Build history of the part. All positions in model axes, mm. Face numbers are marked on the shaded views. A direction names the side the tool comes from. Give positions to 0.01 mm unless a question says otherwise; leave off trailing zeros. Order: outer loops, then holes, each group sorted by start corner. A loop starts at its lowest first (then second) coordinate and runs counter-clockwise, first axis right, second up. Notation, with made-up numbers: (36.5, 1) - (72.5, 1) arc R31 ccw to (72.5, 25) - close; hole circle Ø6 at (-11, 30). An arc over 180 degrees is marked (long way). Answer in a Markdown table with one row per item.
```python
from build123d import *

# Parameters (mm, degrees)
F0_R     = 15
F1_DEPTH = 15
F3_DEPTH = 10
F4_R     = 6
F5_DEPTH = 10


with BuildPart() as f1:
    # F0 (on Top) → F1 (new body)
    with BuildSketch(Plane.XY):
        Circle(F0_R)
    extrude(amount=-F1_DEPTH)

    # F2 (on Top) → F3 (cut, symmetric)
    with BuildSketch(Plane.XY):
        Polygon((4.235221, 4.27539), (-15.764779, 4.27539), (-15.764779, 0.07539), (-0.001056, 0.035212), (-0.001056, -19.964788), (4.198944, -19.964788), align=None)
    extrude(amount=F3_DEPTH, both=True, mode=Mode.SUBTRACT)

    # F4 (on Top) → F5 (cut, symmetric)
    with BuildSketch(Plane.XY):
        with Locations((2.316362, 1.923726)):
            Circle(F4_R)
    extrude(amount=F5_DEPTH, both=True, mode=Mode.SUBTRACT)


solid = f1.part
```
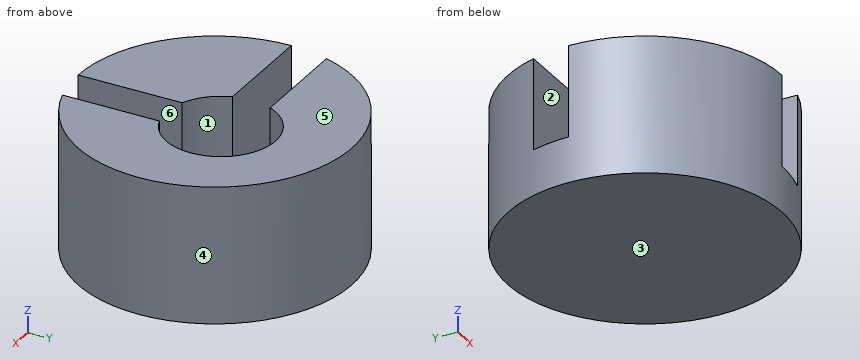
1. Drop flat-ended pins along their axis: P1, Ø1, axis at x = 10.5, y = 7, coming from the +Z side; P2, Ø5, axis at y = -7.5, z = -7, coming from the +X side; P3, Ø2, axis at y = 10.5, z = -12, coming from the -X side; P4, Ø1.5, axis at x = 10, z = -11, coming from the -Y side. Give the stop position or say it passes through.
Check result:
| item | result |
|---|---|
| P1 | stops at z = 0 |
| P2 | stops at x = 14.14 |
| P3 | stops at x = -11.61 |
| P4 | stops at y = -11.81 |
2. Cut at A-A on z = -7.25. Write the cut outline in (x, y).
Check result:
| item | result |
|---|---|
| outline | (-15, 0.07) arc R15 ccw to (0, -15) - (0, -3.61) arc R6 cw to (-3.38, 0.04) - close; (-14.38, 4.28) - (-3.2, 4.28) arc R6 cw (long way) to (4.22, -3.77) - (4.21, -14.4) arc R15 ccw (long way) to start |
3. Two-plate mould, pull along X, no slides. Class the marked faces 4, 5 and 6: +X half, -X half, draft (parallel to the pull), parting line (faces both ways), or undercut.
Check result:
| item | result |
|---|---|
| face 4 | parting line |
| face 5 | draft |
| face 6 | undercut |
4. Cut at B-B on x = -5. Write the cut outline in (y, z), and give its area (3 significant figures).
Check result:
| item | result |
|---|---|
| outline | (-14.14, -15) - (14.14, -15) - (14.14, 0) - (4.28, 0) - (4.28, -10) - (0.05, -10) - (0.05, 0) - (-14.14, 0) - close |
| area | 382 mm² |
5. Cut at C-C on y = -13. Write the cut outline in (x, z), and give its area (3 significant figures).
Check result:
| item | result |
|---|---|
| outline | (-7.48, -15) - (7.48, -15) - (7.48, 0) - (4.21, 0) - (4.21, -10) - (0, -10) - (0, 0) - (-7.48, 0) - close |
| area | 182 mm² |
6. Which spindle directions (+Z, -Z, +X, -X, +Y, -Y) get a long thin tool onto all of the face, cutting with end or side? Do the marked faces 1, 2 and 3. Say none if no direction does.
Check result:
| item | result |
|---|---|
| face 1 | +Z |
| face 2 | +Z, -X |
| face 3 | -Z, +X, -X, +Y, -Y |
7. Probe line 1 (Z direction, x = 6.75, y = 2.75); line 2 (X direction, y = -9.75, z = -9.25); line 3 (Y direction, x = -10.5, z = -6.25). List the from-to ranges inside material, lowest first.
Check result:
| item | result |
|---|---|
| line 1 | z = -15 to -10 |
| line 2 | x = -11.4 to 0, 4.21 to 11.4 |
| line 3 | y = -10.71 to 0.06, 4.28 to 10.71 |
8. Cut at D-D on z = -13.5. Write the cut outline in (x, y), and give its area (3 significant figures).
Check result:
| item | result |
|---|---|
| outline | circle Ø30 at (0, 0) |
| area | 707 mm² |
